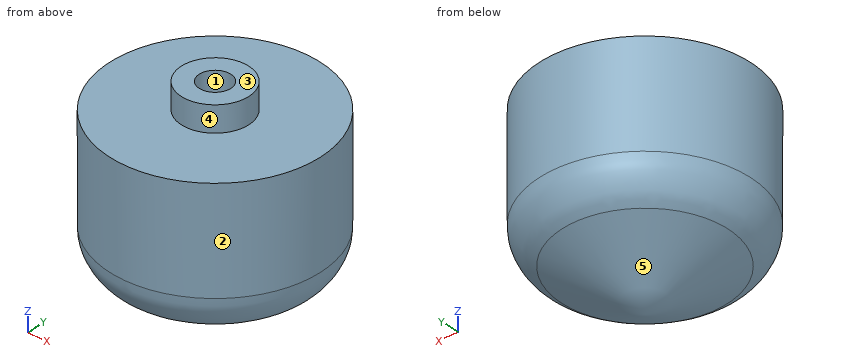
from build123d import *

# Parameters (mm, degrees)
F2_R     = 4.7625
F3_DEPTH = 9.525
F5_R     = 12.7


# Not quite as in the source:
# - the program builds the solid bodies; features that only make, move or delete a surface that nothing else refers to are left out


with BuildPart() as f1:
    # F0 (on Front) → F1 (revolve)
    with BuildSketch(Plane.XZ):
        Polygon((10.16, 55.7645447552), (10.16, 63.5), (0, 63.5), (0, 0), (31.75, 16.6865773499), (31.75, 28.8652195452), (31.75, 46.2049523592), (31.75, 55.7645447552), align=None)
    revolve(axis=Axis((0, 0, 31.75), (0, 0, -1)))

    # F2 (on face) → F3 (cut)
    with BuildSketch(Plane.XY.offset(63.5)):
        Circle(F2_R)
    extrude(amount=-F3_DEPTH, mode=Mode.SUBTRACT)

    # F5
    f5_edges = [f1.edges().sort_by_distance(p)[0] for p in [
        (-31.75, 0, 16.686577),
    ]]
    fillet(f5_edges, radius=F5_R)


solid = f1.part
Geometry: final body of the model. Coordinates: model frame, mm. Face numbers are marked on the shaded views. A direction names the side the tool comes from. Give positions to 0.01 mm unless a question says otherwise; leave off trailing zeros. Write each loop counter-clockwise with the first axis right and the second up, starting at its lowest first coordinate (ties: lowest second). Pieces come first, ordered by that corner, then holes.
(1) Access query for the marked faces 4 and 5. Directions: +Z, -Z, +X, -X, +Y, -Y. A direction counts if a zero-diameter tool reaches every point of the face in a straight line with its end or side. Return the directions, or none.
(2) Cut plane A-A, the plane z = 38.5. Return loops of the section in (x, y), then the cut area to 3 significant figures.
(3) Ray query, line 1 (Y direction, x = 0, z = 56); line 2 (Z direction, x = 11, y = 21); line 3 (Z direction, x = -13, y = -16). Return the intervals inside material, ascending.
(4) First-contact query: P1, Ø7.5, axis at x = 0, y = 0, coming from the -Z side; P2, Ø2, axis at y = -6, z = 9.5, coming from the +X side; P3, Ø10, axis at y = 17.5, z = 9.5, coming from the -X side; P4, Ø10, axis at x = -12.5, y = -4.5, coming from the -Z side. Flat tips, straight axial feed; report the tip coordinate or a pass-through.
(5) Mould query, pull axis X, two halves, no side actions, for the marked faces 1, 2 and 3. Classes: released by +X, released by -X, zero draft, split by the parting line, or undercut.
(6) Cut plane B-B, the plane z = 7. Return loops of the section in (x, y), then the cut area to 3 significant figures.
Values follow:
1. face 4: +Z
1. face 5: -Z
2. outline: circle Ø63.5 at (0, 0)
2. area: 3,170 mm2
3. line 1: y = -10.16 to -4.76, 4.76 to 10.16
3. line 2: z = 12.46 to 55.76
3. line 3: z = 10.83 to 55.76
4. P1: stops at z = 0
4. P2: stops at x = 19.08
4. P3: stops at x = -21.51
4. P4: stops at z = 4.35
5. face 1: undercut
5. face 2: split by the parting line
5. face 3: zero draft
6. outline: circle Ø26.64 at (0, 0)
6. area: 557 mm2
